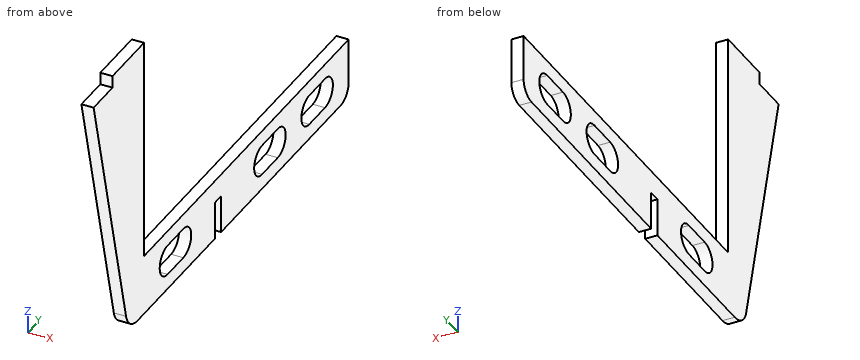
Autodesk Inventor part; units mm, degrees
ref_plane "YZ Plane" through (0, 0, 0) normal (1, 0, 0) x (0, 1, 0)
ref_plane "XZ Plane" through (0, 0, 0) normal (0, 1, 0) x (-1, 0, 0)
ref_plane "XY Plane" through (0, 0, 0) normal (0, 0, 1) x (1, 0, 0)
sketch "Sketch1" plane through (0, 0, 0) normal (1, 0, 0) x (0, 1, 0)
  line L0 (0, 0) -> (50.8, 0)
  line L1 (50.8, 0) -> (50.8, -187.96)
  line L2 (50.8, -187.96) -> (381, -187.96)
  line L3 (381, -187.96) -> (381, -226.06)
  line L4 (0, 0) -> (0, -10.16)
  line L5 (0, -10.16) -> (-30.48, -10.16)
  line L6 (-30.48, -10.16) -> (21.8491, -224.2335)
  line L7 (40.3542, -238.76) -> (368.3, -238.76)
  line L8 (342.9, -200.66) -> (317.5, -200.66)
  line L9 (304.8, -213.36) -> (304.8, -213.36)
  line L10 (317.5, -226.06) -> (342.9, -226.06)
  line L11 (355.6, -213.36) -> (355.6, -213.36)
  line L12 (266.7, -200.66) -> (241.3, -200.66)
  line L13 (228.6, -213.36) -> (228.6, -213.36)
  line L14 (241.3, -226.06) -> (266.7, -226.06)
  line L15 (279.4, -213.36) -> (279.4, -213.36)
  line L16 (152.4, -213.36) -> (152.4, -213.36)
  line L17 (203.2, -213.36) -> (203.2, -213.36)
  line L18 (114.3, -200.66) -> (88.9, -200.66)
  line L19 (76.2, -213.36) -> (76.2, -213.36)
  line L20 (88.9, -226.06) -> (114.3, -226.06)
  line L21 (127, -213.36) -> (127, -213.36)
  line L22 (127, -226.06) -> (152.4, -226.06)
  line L23 (203.2, -226.06) -> (228.6, -226.06)
  line L24 (279.4, -226.06) -> (304.8, -226.06)
  line L25 (355.6, -226.06) -> (381, -226.06)
  line L26 (355.6, -226.06) -> (355.6, -238.76)
  arc A0 (355.6, -213.36) -> (342.9, -200.66) centre (342.9, -213.36) ccw
  arc A1 (342.9, -226.06) -> (355.6, -213.36) centre (342.9, -213.36) ccw
  arc A2 (317.5, -200.66) -> (304.8, -213.36) centre (317.5, -213.36) ccw
  arc A3 (304.8, -213.36) -> (317.5, -226.06) centre (317.5, -213.36) ccw
  arc A4 (279.4, -213.36) -> (266.7, -200.66) centre (266.7, -213.36) ccw
  arc A5 (266.7, -226.06) -> (279.4, -213.36) centre (266.7, -213.36) ccw
  arc A6 (241.3, -200.66) -> (228.6, -213.36) centre (241.3, -213.36) ccw
  arc A7 (228.6, -213.36) -> (241.3, -226.06) centre (241.3, -213.36) ccw
  arc A8 (127, -213.36) -> (114.3, -200.66) centre (114.3, -213.36) ccw
  arc A9 (88.9, -200.66) -> (76.2, -213.36) centre (88.9, -213.36) ccw
  arc A10 (76.2, -213.36) -> (88.9, -226.06) centre (88.9, -213.36) ccw
  arc A11 (114.3, -226.06) -> (127, -213.36) centre (114.3, -213.36) ccw
  arc A12 (21.8491, -224.2335) -> (40.3542, -238.76) centre (40.3542, -219.71) ccw
  arc A13 (368.3, -238.76) -> (381, -226.06) centre (368.3, -226.06) ccw
  line L27 (165.1, -238.76) -> (165.1, -207.01)
  line L28 (165.1, -207.01) -> (175.26, -207.01)
  line L29 (175.26, -207.01) -> (175.26, -238.76)
  point P0 (381, -238.76)
  point P1 (355.6, -200.66)
  point P2 (279.4, -200.66)
  point P3 (203.2, -200.66)
  point P4 (127, -200.66)
  point P5 (76.2, -226.06)
  point P6 (127, -213.36)
  point P7 (76.2, -213.36)
  point P8 (228.6, -213.36)
  point P9 (355.6, -213.36)
  point P10 (304.8, -213.36)
  dimension "d0" = 50.8
  dimension "d1" = 187.96
  dimension "d2" = 330.2
  dimension "d3" = 50.8
  dimension "d5" = 10.16
  dimension "d6" = 30.48
  dimension "d10" = 50.8
  dimension "d11" = 25.4
  dimension "d12" = 25.4
  dimension "d13" = 12.7
  dimension "d14" = 12.7
  dimension "d15" = 50.8
  dimension "d16" = 50.8
  dimension "d17" = 50.8
  dimension "d18" = 12.7
  dimension "d19" = 19.05
  dimension "d22" = 12.7
  dimension "d24" = 12.7
  dimension "d25" = 10.16
  dimension "d26" = 31.75
  dimension "d27" = 114.3
  dimension "d28" = 196.85
extrude "Extrusion1" add sketch "Sketch1" along normal blind 10.16 contours L0 L1 L2 L3 L25 L26 L7 L29 L28 L27 A12 L6 L5 L4 | A13 L7 L26 L25
properties part number "battery front brace"
Here's how the part is built. I have some questions about the finished solid (model axes, mm). Round coordinates to 2 decimals unless told otherwise and drop trailing zeros. Order: outer loops, then holes, each group sorted by start corner. A loop starts at its lowest first (then second) coordinate and runs counter-clockwise, first axis right, second up. Notation, with made-up numbers: M 55.25,55.25 L 91.25,55.25 A15 ccw 91.25,73.25 Z; hole C -35.5,85.25 d9. An arc over 180 degrees is marked long. One line per question, with ' | ' between items.
1) I need wall thicknesses on line 1 along Z through (x, y) = (1.25, 321.5); line 2 along Z through (x, y) = (5.25, 156.5); line 3 along Y through (x, z) = (5, -202). Which ranges of each line are inside material? Lowest first, please.
Working result:
line 1: -238.76 to -226.06, -200.66 to -187.96 | line 2: -238.76 to -187.96 | line 3: 16.41 to 83.22, 119.98 to 235.62, 272.38 to 311.82, 348.58 to 381
2) For pin 1 Ø3 at (x, z) = (5, -217) entering from -Y; pin 2 Ø1.5 at (x, y) = (7.5, 294) entering from +Z; pin 3 Ø1.5 at (x, z) = (6, -36.5) entering from +Y, each with a flat end and sliding along its axis, tell me the tip position at first contact or that it passes through.
Working result:
pin 1: y = 19.71 | pin 2: z = -187.96 | pin 3: y = 50.8
3) I want a section at A-A, the plane z = -213.36. Write out the boundary of the cut face in (x, y).
Working result:
outline: M 0,19.19 L 10.16,19.19 L 10.16,76.2 L 0,76.2 Z; M 0,127 L 10.16,127 L 10.16,165.1 L 0,165.1 Z; M 0,175.26 L 10.16,175.26 L 10.16,228.6 L 0,228.6 Z; M 0,279.4 L 10.16,279.4 L 10.16,304.8 L 0,304.8 Z; M 0,355.6 L 10.16,355.6 L 10.16,381 L 0,381 Z
4) I want a section at B-B, the plane y = 207. Write out the boundary of the cut face in (x, z), then the cut area to 3 significant figures.
Working result:
outline: M 0,-238.76 L 10.16,-238.76 L 10.16,-187.96 L 0,-187.96 Z | area: 516 mm²
5) I want a section at C-C, the plane z = -105.5. Write out the boundary of the cut face in (x, y).
Working result:
outline: M 0,-7.17 L 10.16,-7.17 L 10.16,50.8 L 0,50.8 Z
